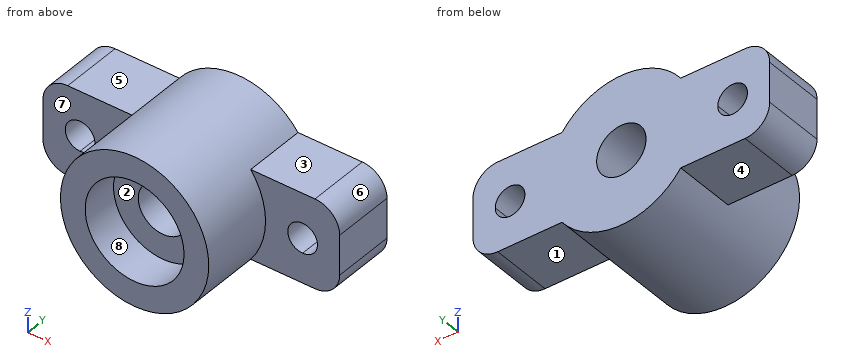
```python
from build123d import *

# Parameters (mm, degrees)
F0_R     = 10
F1_DEPTH = 25
F2_R     = 30
F2_R_2   = 10
F3_DEPTH = 15
F4_R     = 30
F4_R_2   = 20
F5_DEPTH = 15


with BuildPart() as f1:
    # F0 (on Front) → F1 (new body)
    with BuildSketch(Plane.XZ):
        with BuildLine():
            ThreePointArc((24, -18), (28.4604989415, -9.4868329805), (30, 0))
            ThreePointArc((30, 0), (28.4604989415, 9.4868329805), (24, 18))
            Line((24, 18), (-24, 18))
            ThreePointArc((-24, 18), (-30, 0), (-24, -18))
            Line((-24, -18), (24, -18))
        make_face()
        Circle(F0_R, mode=Mode.SUBTRACT)
        with BuildLine():
            ThreePointArc((24, 18), (28.4604989415, 9.4868329805), (30, 0))
            ThreePointArc((30, 0), (28.4604989415, -9.4868329805), (24, -18))
            Line((24, -18), (45, -18))
            Line((45, -18), (50, -18))
            ThreePointArc((50, -18), (57.0710678119, -15.0710678119), (60, -8))
            Line((60, -8), (60, 8))
            ThreePointArc((60, 8), (57.0710678119, 15.0710678119), (50, 18))
            Line((50, 18), (24, 18))
        make_face()
        with BuildLine():
            ThreePointArc((51, 0), (49.2426406871, -4.2426406871), (45, -6))
            ThreePointArc((45, -6), (40.7573593129, 4.2426406871), (51, 0))
        make_face(mode=Mode.SUBTRACT)
        with BuildLine():
            Line((-24, 18), (24, 18))
            ThreePointArc((24, 18), (0, 30), (-24, 18))
        make_face()
        with BuildLine():
            ThreePointArc((-24, -18), (0, -30), (24, -18))
            Line((24, -18), (-24, -18))
        make_face()
        with BuildLine():
            ThreePointArc((-24, -18), (-30, 0), (-24, 18))
            Line((-24, 18), (-50, 18))
            ThreePointArc((-50, 18), (-57.0710678119, 15.0710678119), (-60, 8))
            Line((-60, 8), (-60, -8))
            ThreePointArc((-60, -8), (-57.0710678119, -15.0710678119), (-50, -18))
            Line((-50, -18), (-45, -18))
            Line((-45, -18), (-24, -18))
        make_face()
        with BuildLine():
            ThreePointArc((-39, 0), (-40.7573593129, -4.2426406871), (-45, -6))
            ThreePointArc((-45, -6), (-49.2426406871, 4.2426406871), (-39, 0))
        make_face(mode=Mode.SUBTRACT)
    extrude(amount=F1_DEPTH)

    # F2 (on face) → F3 (join)
    with BuildSketch(Plane.XZ.offset(25)):
        Circle(F2_R)
        Circle(F2_R_2, mode=Mode.SUBTRACT)
    extrude(amount=F3_DEPTH)

    # F4 (on face) → F5 (join)
    with BuildSketch(Plane.XZ.offset(40)):
        Circle(F4_R)
        Circle(F4_R_2, mode=Mode.SUBTRACT)
    extrude(amount=F5_DEPTH)


solid = f1.part
```
Check sheet for the modelled part. Datum: model origin and axes. Units: mm. Face numbers are marked on the shaded views. A direction names the side the tool comes from. Give positions to 0.01 mm unless a question says otherwise; leave off trailing zeros. Write each loop counter-clockwise with the first axis right and the second up, starting at its lowest first coordinate (ties: lowest second). Pieces come first, ordered by that corner, then holes. Notation, with made-up numbers: (85.25, 77.5) -> (101.25, 77.5) arc R20 cw to (101.25, 87.5) -> close; hole circle Ø4 at (66, 60). An arc over 180 degrees is marked (long way). Use CSV: the item, a comma, the result in double quotes. Start each with the question number.
Q1. Cross-section at C-C on y = -27.5. Enter the section's corners in (x, z), and give its area (3 significant figures).
Q2. Cross-section at B-B on x = 47. Enter the section's corners in (y, z).
Q3. Cross-section at A-A on y = -6.5. Enter the section's corners in (x, z), and give its area (3 significant figures).
Q4. Depth check by flat-ended pin: P1, Ø12.5, axis at x = -32, y = -18, coming from the +Z side; P2, Ø19, axis at x = -45, z = 0, coming from the +Y side; P3, Ø8, axis at x = 5.5, y = -47, coming from the -Z side; P4, Ø5, axis at y = -29.5, z = -22.5, coming from the +X side. Enter the tip coordinate at first touch or a pass-through.
Q5. Release check for a two-part mould opening along X. For the marked faces 6, 7 and 8 record: +X half, -X half, draft (parallel to the pull), parting line (faces both ways), or undercut.
Q6. Scan lines: line 1 along Z through (x, y) = (0, -46.25); line 2 along Z through (x, y) = (45, -12.5); line 3 along Z through (x, y) = (30, -9). Record each from-to range of solid material in increasing order.
Q7. Cross-section at D-D on x = 18.5. Enter the section's corners in (y, z), and give its area (3 significant figures).
Q8. Tool access check on the marked faces 1, 2, 3, 4 and 5. Record the directions out of +Z, -Z, +X, -X, +Y, -Y that give a thin tool (end or side, any length) a straight path to the whole face; none if there is none.
Working result:
1,outline,"circle Ø60 at (0, 0); hole circle Ø20 at (0, 0)"
1,area,"2,510 mm^2"
2,outline,"(-25, -18) -> (0, -18) -> (0, -5.66) -> (-25, -5.66) -> close; (-25, 5.66) -> (0, 5.66) -> (0, 18) -> (-25, 18) -> close"
3,outline,"(-60, -8) arc R10 ccw to (-50, -18) -> (-24, -18) arc R30 ccw to (24, -18) -> (50, -18) arc R10 ccw to (60, -8) -> (60, 8) arc R10 ccw to (50, 18) -> (24, 18) arc R30 ccw to (-24, 18) -> (-50, 18) arc R10 ccw to (-60, 8) -> close; hole circle Ø12 at (-45, 0); hole circle Ø20 at (0, 0); hole circle Ø12 at (45, 0)"
3,area,"4,500 mm^2"
4,P1,"stops at z = 18"
4,P2,"stops at y = 0"
4,P3,"stops at z = -29.96"
4,P4,"stops at x = 22.36"
5,face 6,"+X half"
5,face 7,"draft"
5,face 8,"undercut"
6,line 1,"z = -30 to -20, 20 to 30"
6,line 2,"z = -18 to -6, 6 to 18"
6,line 3,"z = -18 to 18"
7,outline,"(-55, -23.62) -> (0, -23.62) -> (0, 23.62) -> (-55, 23.62) -> (-55, 7.6) -> (-40, 7.6) -> (-40, -7.6) -> (-55, -7.6) -> close"
7,area,"2,370 mm^2"
8,face 1,"-Z, +X, +Y, -Y"
8,face 2,"-Y"
8,face 3,"+Z, +X, +Y, -Y"
8,face 4,"-Z, -X, +Y, -Y"
8,face 5,"+Z, -X, +Y, -Y"
